CAD build for the part. Positions are in the model's coordinates, mm. A direction names the side the tool comes from. Round coordinates to 2 decimals unless told otherwise and drop trailing zeros. Write each loop counter-clockwise with the first axis right and the second up, starting at its lowest first coordinate (ties: lowest second). Pieces come first, ordered by that corner, then holes. Notation, with made-up numbers: (-4.5, -13) - (8.5, -13) arc R17 cw to (8.5, 3) - close; hole circle Ø7 at (2.5, 38). An arc over 180 degrees is marked (long way). Put each result on its own line as item: value. Start each with the question number.
Item 1: 3-axis set-ups, long thin cutter, end or side, ignore diameter. For faces 1 (the flat face through (-1, 1, 0)), 2 (the flat face through (1, -61.75, 11)): which of +Z, -Z, +X, -X, +Y, -Y reach the whole face in a straight line?
Item 2: Cut at A-A (z = 8). Give the cut face in (x, y).
Item 3: Cut at C-C (x = 34.5). Give the cut face in (y, z), and give its area (3 significant figures).
Item 4: Cut at B-B (y = -10.5). Give the cut face in (x, z).
Item 5: Mould opens along X. For faces 3 (the cylindrical face through (-94.25, 61.32, 9.86)), 4 (the flat face through (-1, -62.75, 10)), 5 (the flat face through (-1, 1, 2)) say: released by +X, released by -X, zero draft, split by the parting line, or undercut.
Item 6: Drill centre lines: line 1 (Y direction, x = 69.5, z = 10.75); line 2 (X direction, y = 33, z = 12.5); line 3 (Z direction, x = -41, y = -42.5). Where is each one in solid material? Low to high. Write a range as from..to.
```python
from build123d import *

# Parameters (mm, degrees)
F1_DEPTH = 20
F3_DEPTH = 2


with BuildPart() as f1:
    # F0 (on Top) → F1 (new body)
    with BuildSketch(Plane.XY):
        with BuildLine():
            ThreePointArc((95.75, 57.75), (94.285534, 61.285534), (90.75, 62.75))
            Line((90.75, 62.75), (-90.75, 62.75))
            ThreePointArc((-90.75, 62.75), (-94.285534, 61.285534), (-95.75, 57.75))
            Line((-95.75, 57.75), (-95.75, -57.75))
            ThreePointArc((-95.75, -57.75), (-94.285534, -61.285534), (-90.75, -62.75))
            Line((-90.75, -62.75), (90.75, -62.75))
            ThreePointArc((90.75, -62.75), (94.285534, -61.285534), (95.75, -57.75))
            Line((95.75, -57.75), (95.75, 57.75))
        make_face()
        with BuildLine():
            Line((-89.75, 61.75), (89.75, 61.75))
            ThreePointArc((89.75, 61.75), (93.285534, 60.285534), (94.75, 56.75))
            Line((94.75, 56.75), (94.75, -56.75))
            ThreePointArc((94.75, -56.75), (93.285534, -60.285534), (89.75, -61.75))
            Line((89.75, -61.75), (-89.75, -61.75))
            ThreePointArc((-89.75, -61.75), (-93.285534, -60.285534), (-94.75, -56.75))
            Line((-94.75, -56.75), (-94.75, 56.75))
            ThreePointArc((-94.75, 56.75), (-93.285534, 60.285534), (-89.75, 61.75))
        make_face(mode=Mode.SUBTRACT)
    extrude(amount=F1_DEPTH)

    # F2 (on Top) → F3 (join)
    with BuildSketch(Plane.XY):
        with BuildLine():
            ThreePointArc((95.75, 57.75), (94.285534, 61.285534), (90.75, 62.75))
            Line((90.75, 62.75), (-90.75, 62.75))
            ThreePointArc((-90.75, 62.75), (-94.285534, 61.285534), (-95.75, 57.75))
            Line((-95.75, 57.75), (-95.75, -57.75))
            ThreePointArc((-95.75, -57.75), (-94.285534, -61.285534), (-90.75, -62.75))
            Line((-90.75, -62.75), (90.75, -62.75))
            ThreePointArc((90.75, -62.75), (94.285534, -61.285534), (95.75, -57.75))
            Line((95.75, -57.75), (95.75, 57.75))
        make_face()
    extrude(amount=F3_DEPTH)


solid = f1.part
```
Output values:
1. face 1: -Z, +X, -X, +Y, -Y
1. face 2: +Z
2. outline: (-95.75, -57.75) arc R5 ccw to (-90.75, -62.75) - (90.75, -62.75) arc R5 ccw to (95.75, -57.75) - (95.75, 57.75) arc R5 ccw to (90.75, 62.75) - (-90.75, 62.75) arc R5 ccw to (-95.75, 57.75) - close; hole (-94.75, -56.75) arc R5 ccw to (-89.75, -61.75) - (89.75, -61.75) arc R5 ccw to (94.75, -56.75) - (94.75, 56.75) arc R5 ccw to (89.75, 61.75) - (-89.75, 61.75) arc R5 ccw to (-94.75, 56.75) - close
3. outline: (-62.75, 0) - (62.75, 0) - (62.75, 20) - (61.75, 20) - (61.75, 2) - (-61.75, 2) - (-61.75, 20) - (-62.75, 20) - close
3. area: 287 mm2
4. outline: (-95.75, 0) - (95.75, 0) - (95.75, 20) - (94.75, 20) - (94.75, 2) - (-94.75, 2) - (-94.75, 20) - (-95.75, 20) - close
5. face 3: released by -X
5. face 4: zero draft
5. face 5: undercut
6. line 1: -62.75..-61.75, 61.75..62.75
6. line 2: -95.75..-94.75, 94.75..95.75
6. line 3: 0..2
